```python
from build123d import *

# Parameters (mm, degrees)
SKETCH1_W                  = 88.9
SKETCH1_H                  = 63.5
BOSS_EXTRUDE1_DEPTH        = 12.7
SKETCH2_W                  = 57.15
SKETCH2_H                  = 7.9375
CUT_EXTRUDE1_DEPTH         = 79.545162168
F_10_24_TAPPED_HOLE1_D     = 3.7973
CUT_EXTRUDE2_DEPTH         = 25.4
BOSS_EXTRUDE2_START        = 44.45
BOSS_EXTRUDE2_DEPTH        = 7.9375
BOSS_EXTRUDE3_START        = -36.5125
BOSS_EXTRUDE3_DEPTH        = 7.9375
SKETCH7_W                  = 73.025
SKETCH7_H                  = 89.79384994
BOSS_EXTRUDE4_DEPTH        = 7.9375
SKETCH8_R                  = 15.875
SKETCH8_R_2                = 7.9375
BOSS_EXTRUDE5_DEPTH        = 57.15
F_10_24_TAPPED_HOLE2_D     = 3.7973
F_10_24_TAPPED_HOLE2_DEPTH = 15.875


with BuildPart() as part:
    # Sketch1 → Boss-Extrude1 (new, symmetric)
    with BuildSketch(Plane(origin=(0, 0, 0), x_dir=(1, 0, 0), z_dir=(0, 1, 0))):
        Rectangle(SKETCH1_W, SKETCH1_H)
    extrude(amount=BOSS_EXTRUDE1_DEPTH, both=True)

    # Sketch2 → Cut-Extrude1 (cut, through all)
    with BuildSketch(Plane.XY.offset(31.75)):
        with Locations((0, -8.73125)):
            Rectangle(SKETCH2_W, SKETCH2_H)
    extrude(amount=-CUT_EXTRUDE1_DEPTH, mode=Mode.SUBTRACT)

    # #10-24 Tapped Hole1 (through all)
    with Locations(Plane.XY.offset(31.75)):
        with Locations((-3.175, 3.96875)):
            Hole(F_10_24_TAPPED_HOLE1_D / 2)

    # Sketch5 → Cut-Extrude2 (cut)
    with BuildSketch(Plane(origin=(0, 12.7, 0), x_dir=(1, 0, 0), z_dir=(0, 1, 0))):
        with BuildLine():
            Line((-7.9375, -19.05), (-7.9375, 6.35))
            ThreePointArc((-7.9375, 6.35), (-3.175, 11.1125), (1.5875, 6.35))
            Line((1.5875, 6.35), (1.5875, -19.05))
            ThreePointArc((1.5875, -19.05), (-3.175, -23.8125), (-7.9375, -19.05))
        make_face()
    extrude(amount=-CUT_EXTRUDE2_DEPTH, mode=Mode.SUBTRACT)

    # Sketch6 → Boss-Extrude2 (add)
    with BuildSketch(Plane(origin=(0, 0, 0), x_dir=(0, 0, -1), z_dir=(1, 0, 0)).offset(BOSS_EXTRUDE2_START)):
        with BuildLine():
            Line((-31.75, 12.7), (-19.267674347, 99.045324328))
            ThreePointArc((-19.267674347, 99.045324328), (-2.928920422, 80.911389994), (11.927343936, 100.278523586))
            Line((11.927343936, 100.278523586), (31.75, 12.7))
            Line((31.75, 12.7), (-31.75, 12.7))
        make_face()
    extrude(amount=-BOSS_EXTRUDE2_DEPTH)

    # Sketch6<2> → Boss-Extrude3 (add)
    with BuildSketch(Plane(origin=(0, 0, 0), x_dir=(0, 0, -1), z_dir=(1, 0, 0)).offset(BOSS_EXTRUDE3_START)):
        with BuildLine():
            Line((-31.75, 12.7), (-19.267674347, 99.045324328))
            ThreePointArc((-19.267674347, 99.045324328), (-2.928920422, 80.911389994), (11.927343936, 100.278523586))
            Line((11.927343936, 100.278523586), (31.75, 12.7))
            Line((31.75, 12.7), (-31.75, 12.7))
        make_face()
    extrude(amount=-BOSS_EXTRUDE3_DEPTH)

    # Sketch7 → Boss-Extrude4 (add)
    with BuildSketch(Plane(origin=(0, 7.455044818, -32.937151123), x_dir=(-1, 0, 0), z_dir=(0, 0.22075739126394447, -0.9753287518587453))):
        with Locations((0, 50.274552946)):
            Rectangle(SKETCH7_W, SKETCH7_H)
    extrude(amount=-BOSS_EXTRUDE4_DEPTH)

    # Sketch8 → Boss-Extrude5 (add, symmetric)
    with BuildSketch(Plane(origin=(0, 0, 0), x_dir=(0, 0, -1), z_dir=(1, 0, 0))):
        with Locations((-3.556, 96.774)):
            Circle(SKETCH8_R)
        with Locations((-3.556, 96.774)):
            Circle(SKETCH8_R_2, mode=Mode.SUBTRACT)
    extrude(amount=BOSS_EXTRUDE5_DEPTH, both=True)

    # #10-24 Tapped Hole2
    with Locations(Plane(origin=(44.45, 0, 0), x_dir=(0, 0, -1), z_dir=(1, 0, 0))):
        with Locations((-15.875, -8.73125), (15.875, -8.73125)):
            Hole(F_10_24_TAPPED_HOLE2_D / 2, depth=F_10_24_TAPPED_HOLE2_DEPTH)


solid = part.part
```
CAD build for the part. Positions are in the model's coordinates, mm. A direction names the side the tool comes from. Give positions to 0.01 mm unless a question says otherwise; leave off trailing zeros. Loops run counter-clockwise (first coordinate to the right, second up) from the corner with the lowest first, then second, coordinate; pieces in that order, holes last. Notation, with made-up numbers: (48, 33) - (59, 33) arc R19 cw to (59, 38) - close; hole circle Ø9 at (85.25, 31.25). An arc over 180 degrees is marked (long way). Put each result on its own line as item: value.
Q1. Tool access for faces 1 (the face through (-3.28, 6.03, -11.11)), 2 (the face through (-28.575, -9, 0)), 3 (the face through (-37, -12.7, 0)): list every direction of +Z, -Z, +X, -X, +Y, -Y with a clear straight run to the whole face (end or side of a thin tool).
Filled in:
face 1: -Y
face 2: +Z, -Z, -Y
face 3: +Z, -Z, +X, -X, -Y
Q2. Mould opens along Y. For faces 4 (the face through (40.537, 55.268, 25.596)), 5 (the face through (-1, 3, 31.75)), 6 (the face through (36.512, 47, 4)) say: pulls with the +Y half, pulls with the -Y half, needs draft (parallel to the pull), parting line crosses it, or undercut.
Filled in:
face 4: pulls with the +Y half
face 5: needs draft
face 6: undercut
Q3. Slice it at D-D (y = 25.5). Give the cut face in (x, z), plus the area to 3 significant figures.
Filled in:
outline: (-44.45, -28.85) - (44.45, -28.85) - (44.45, 29.9) - (36.51, 29.9) - (36.51, -20.71) - (-36.51, -20.71) - (-36.51, 29.9) - (-44.45, 29.9) - close
area: 1,530 mm²
Q4. Probe line 1 along X through (y, z) = (36.5, -9.5); line 2 along Y through (x, z) = (-36, 5.5). List the from-to ranges inside material, lowest first.
Filled in:
line 1: x = -44.45 to -36.51, 36.51 to 44.45
line 2: y = -12.7 to 12.7, 81.02 to 89.08, 104.47 to 112.53
Q5. Flat gauge pins, fed straight in: pin 1 (19 mm diameter, centred on y = 2, z = 0, fed in from -X); pin 2 (12.5 mm diameter, centred on y = 96.774, z = 3.556, fed in from -X); pin 3 (3 mm diameter, centred on y = 34, z = -15.5, fed in from +X); pin 4 (8 mm diameter, centred on x = -43.5, y = 63, fed in from +Z). Where does each tip first touch, or does it go through?
Filled in:
pin 1: stops at x = -44.45
pin 2: passes through
pin 3: stops at x = 44.45
pin 4: stops at z = 25.06
Q6. Slice it at C-C (x = 32.5). Give the number of separate pieces and of enclosed holes in the cut face, plus the area to 3 significant figures.
Filled in:
separate pieces: 1
enclosed holes: 3
area: 2,810 mm²
Q7. Slice it at A-A (y = 94). Give the cut face in (x, z), plus the area to 3 significant figures.
Filled in:
outline: (-57.15, -12.07) - (-44.45, -12.07) - (-44.45, -13.35) - (44.45, -13.35) - (44.45, -12.07) - (57.15, -12.07) - (57.15, -3.88) - (-57.15, -3.88) - close; (-57.15, 10.99) - (57.15, 10.99) - (57.15, 19.19) - (44.45, 19.19) - (44.45, 20) - (36.51, 20) - (36.51, 19.19) - (-36.51, 19.19) - (-36.51, 20) - (-44.45, 20) - (-44.45, 19.19) - (-57.15, 19.19) - close
area: 2,000 mm²
